Build history of the part. All positions in model axes, mm. Round coordinates to 2 decimals unless told otherwise and drop trailing zeros. Write each loop counter-clockwise with the first axis right and the second up, starting at its lowest first coordinate (ties: lowest second). Pieces come first, ordered by that corner, then holes. Notation, with made-up numbers: (55, 62) -> (92, 62) arc R13 cw to (92, 76) -> close; hole circle Ø6 at (-31, 57). An arc over 180 degrees is marked (long way). One line per question, with ' | ' between items.
from build123d import *

# Parameters (mm, degrees)
F0_W     = 609.6
F0_H     = 457.2
F0_R     = 6.35
F0_W_2   = 261.167854
F0_H_2   = 39.175182
F1_DEPTH = 3.175


with BuildPart() as f1:
    # F0 (on Front) → F1 (new body)
    with BuildSketch(Plane.XZ):
        with Locations((2.926078, 30.520323)):
            Rectangle(F0_W, F0_H)
        Polygon((-234.366894, -59.028838), (-234.366894, 95.353276), (-220.525727, 95.353276), (-220.525727, -59.028838), (-207.749292, -59.028838), (-207.749292, -151.658103), (-248.208046, -151.658103), (-248.208046, -59.028838), align=None, mode=Mode.SUBTRACT)
        Polygon((-4.236173, -128.238574), (-4.236173, -132.526398), (200.95925, -132.526398), (200.95925, -110.175043), (222.640842, -110.175043), (222.640842, -18.203117), (239.426598, -18.203117), (239.426598, -110.175043), (244.322434, -110.175043), (244.322434, -150.041208), (200.95925, -150.041208), (200.95925, -146.367162), (-4.236173, -146.367162), (-4.236173, -151.014999), (-55.13164, -151.014999), (-55.13164, -128.238574), align=None, mode=Mode.SUBTRACT)
        with BuildLine():
            add(Edge.make_bspline(
                [(-51.138811, 33.683006), (-40.763055, -8.035491), (30.757283, 31.901763), (102.277622, 71.839016), (20.381528, 73.620259), (-61.514566, 75.401502), (-51.138811, 33.683006)],
                knots=[0, 0, 0, 2.094395, 2.094395, 4.18879, 4.18879, 6.283185, 6.283185, 6.283185], degree=2, weights=[1, 0.5, 1, 0.5, 1, 0.5, 1]))
        make_face(mode=Mode.SUBTRACT)
        with Locations((-276.473922, 233.720323)):
            Circle(F0_R, mode=Mode.SUBTRACT)
        with Locations((6.09912, 149.388954)):
            Rectangle(F0_W_2, F0_H_2, mode=Mode.SUBTRACT)
        with Locations((282.326078, 233.720323)):
            Circle(F0_R, mode=Mode.SUBTRACT)
    extrude(amount=F1_DEPTH)


solid = f1.part
(1) Wall check: line 1 (X direction, y = -1.8, z = -132); line 2 (X direction, y = -1.85, z = -57); line 3 (X direction, y = -1.8, z = -118). Give the ranges that are in metal, low to high. Write a range as from..to.
Calculated:
line 1: -301.87..-248.21, -207.75..-55.13, -4.24..200.96, 244.32..307.73 | line 2: -301.87..-234.37, -220.53..222.64, 239.43..307.73 | line 3: -301.87..-248.21, -207.75..200.96, 244.32..307.73
(2) Slice it at C-C (x = 92). Write the cut outline in (y, z) (3 decimals).
Calculated:
outline: (-3.175, -198.08) -> (0, -198.08) -> (0, -146.367) -> (-3.175, -146.367) -> close; (-3.175, -132.526) -> (0, -132.526) -> (0, 129.801) -> (-3.175, 129.801) -> close; (-3.175, 168.977) -> (0, 168.977) -> (0, 259.12) -> (-3.175, 259.12) -> close
(3) Mould opens along Z. For faces 1 (the flat face through (-1, -3.175, -17)), 2 (the cylindrical face through (280.95, -1.57, 227.52)) say: pulls with the +Z half, pulls with the -Z half, needs draft (parallel to the pull), parting line crosses it, or undercut.
Calculated:
face 1: needs draft | face 2: undercut
(4) Slice it at D-D (y = -0.65). State how many separate pieces and enclosed holes the cut face has, then the cut area to 3 significant figures.
Calculated:
separate pieces: 1 | enclosed holes: 6 | area: 251,000 mm2
(5) Slice it at A-A (z = 162). Write the cut outline in (x, y) (3 decimals).
Calculated:
outline: (-301.874, -3.175) -> (-124.485, -3.175) -> (-124.485, 0) -> (-301.874, 0) -> close; (136.683, -3.175) -> (307.726, -3.175) -> (307.726, 0) -> (136.683, 0) -> close
(6) Slice it at B-B (x = -78.5). Write the cut outline in (y, z) (3 decimals), then the cut area to 3 significant figures.
Calculated:
outline: (-3.175, -198.08) -> (0, -198.08) -> (0, 129.801) -> (-3.175, 129.801) -> close; (-3.175, 168.977) -> (0, 168.977) -> (0, 259.12) -> (-3.175, 259.12) -> close | area: 1,330 mm2
